Autodesk Inventor part; units mm, degrees
ref_plane "YZ Plane" through (0, 0, 0) normal (1, 0, 0) x (0, 1, 0)
ref_plane "XZ Plane" through (0, 0, 0) normal (0, 1, 0) x (-1, 0, 0)
ref_plane "XY Plane" through (0, 0, 0) normal (0, 0, 1) x (1, 0, 0)
sketch "Sketch1" plane through (0, 0, 0) normal (0, 0, 1) x (1, 0, 0)
  line L0 (0, 0) -> (25.4, 0)
  line L1 (25.4, 0) -> (25.4, 25.4)
  line L2 (25.4, 25.4) -> (0, 25.4)
  line L3 (0, 25.4) -> (0, 0)
  line L4 (3.175, 22.225) -> (22.225, 22.225)
  line L5 (22.225, 22.225) -> (22.225, 3.175)
  line L6 (22.225, 3.175) -> (3.175, 3.175)
  line L7 (3.175, 3.175) -> (3.175, 22.225)
  dimension "d0" = 25.4
  dimension "d1" = 25.4
  dimension "d2" = 3.175
extrude "Extrusion1" add sketch "Sketch1" against normal blind 590.55
sketch "Sketch3" plane through (25.4, 0, 0) normal (1, 0, 0) x (0, 0, -1)
  line L0 (0, 0) -> (0, 25.4)
  point P0 (203.2, 12.7)
  dimension "d14" = 203.2
hole "Hole2" at (25.4, 12.7, -203.2) direction (-1, 0, 0) diameter 12.7 depth 25.4 tip angle 118
sketch "Sketch4" plane through (0, 0, 0) normal (-1, 0, 0) x (0, 0, 1)
  circle A0 centre (-203.2, 12.7) radius 6.35
  point P0 (-179.3875, 12.7)
  point P1 (-227.0125, 12.7)
  dimension "d23" = 23.8125
  dimension "d24" = 23.8125
hole "Hole3" at (0, 12.7, -179.3875) at (0, 12.7, -227.0125) direction (1, 0, 0) diameter 5.334 depth 25.4 tip angle 118
sketch "Sketch5" plane through (0, 25.4, 0) normal (0, 1, 0) x (1, 0, 0)
  line L0 (25.4, 590.55) -> (0, 590.55)
  line L1 (25.4, 0) -> (0, 0)
  point P0 (12.7, 12.7)
  point P1 (12.7, 38.1)
  point P2 (12.7, 63.5)
  point P3 (12.7, 577.85)
  point P4 (12.7, 552.45)
  dimension "d32" = 12.7
  dimension "d33" = 25.4
  dimension "d34" = 12.7
  dimension "d35" = 25.4
  dimension "d36" = 25.4
hole "Hole4" at (12.7, 25.4, -12.7) at (12.7, 25.4, -38.1) at (12.7, 25.4, -63.5) at (12.7, 25.4, -577.85) at (12.7, 25.4, -552.45) direction (0, -1, 0) diameter 5.334 depth 25.4 tip angle 118
properties part number "new vertical kicker thingleft"
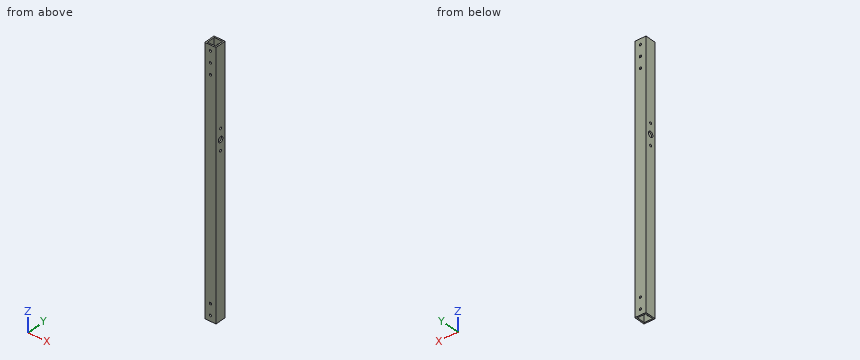
Design review of the part built by this model. Coordinates are the model's own, in mm. Round coordinates to 2 decimals unless told otherwise and drop trailing zeros. Order: outer loops, then holes, each group sorted by start corner. A loop starts at its lowest first (then second) coordinate and runs counter-clockwise, first axis right, second up.
1) Consider section A-A (z = -371.5). State the section outline as (x, y) points (3 decimals).
The answers:
outline: (0, 0) - (25.4, 0) - (25.4, 25.4) - (0, 25.4) - close; hole (3.175, 3.175) - (22.225, 3.175) - (22.225, 22.225) - (3.175, 22.225) - close
2) For L1, parallel to Z at x = 12.7, y = 1; L2, parallel to Z at x = 1.45, y = 12.7; L3, parallel to X at y = 1.15, z = -38.1, list the stretches that pass through material, from the lowest coordinate up.
The answers:
L1: z = -590.55 to -580.52, -575.18 to -555.12, -549.78 to -66.17, -60.83 to -40.77, -35.43 to -15.37, -10.03 to 0
L2: z = -590.55 to -229.68, -224.35 to -209.55, -196.85 to -182.05, -176.72 to 0
L3: x = 0 to 10.03, 15.37 to 25.4
3) Clearance check with a flat-ended pin moving along its axis: pin 1 Ø3 at (y, z) = (12.7, -227.01) entering from +X. State where the tip first meets the part, or that it passes through.
The answers:
pin 1: passes through
